Here's the drawing with two shaded views (mm, measured from the low corner). I have some questions. A direction names the side the tool comes from. Round coordinates to 2 decimals unless told otherwise and drop trailing zeros. Loops run counter-clockwise (first coordinate to the right, second up) from the corner with the lowest first, then second, coordinate; pieces in that order, holes last. Notation, with made-up numbers: (25, 59.5) - (75, 59.5) arc R22 cw to (75, 91.5) - close; hole circle Ø2 at (-15, 32). An arc over 180 degrees is marked (long way). Answer as CSV lines item,"result".
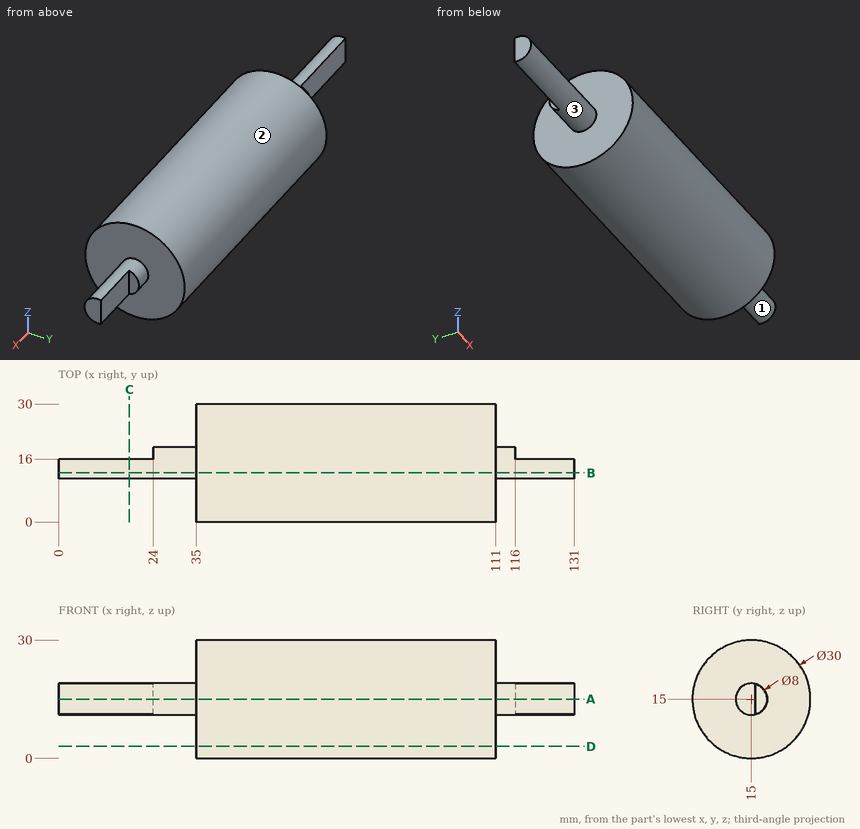
Q1. If I drill on line 1 along X through (y, z) = (7.5, 19.25); line 2 along Y through (x, z) = (103.5, 15.25); line 3 along Z through (x, y) = (8, 14), over which ranges is the centre line in solid material (lowest first)? Write a range as [from, to].
Checks:
line 1,"[35, 111]"
line 2,"[0, 30]"
line 3,"[11.13, 18.87]"
Q2. Imagine slicing it at B-B (y = 12.5). Write out the boundary of the cut face in (x, z).
Checks:
outline,"(0, 11.88) - (35, 11.88) - (35, 0.21) - (111, 0.21) - (111, 11.88) - (131, 11.88) - (131, 18.12) - (111, 18.12) - (111, 29.79) - (35, 29.79) - (35, 18.12) - (0, 18.12) - close"
Q3. Imagine slicing it at A-A (z = 15). Write out the boundary of the cut face in (x, y), then the cut area to 3 significant figures.
Checks:
outline,"(0, 11) - (35, 11) - (35, 0) - (111, 0) - (111, 11) - (131, 11) - (131, 16) - (116, 16) - (116, 19) - (111, 19) - (111, 30) - (35, 30) - (35, 19) - (24, 19) - (24, 16) - (0, 16) - close"
area,"2,600 mm²"
Q4. Imagine slicing it at D-D (z = 3). Write out the boundary of the cut face in (x, y), then the cut area to 3 significant figures.
Checks:
outline,"(35, 6) - (111, 6) - (111, 24) - (35, 24) - close"
area,"1,370 mm²"
Q5. Imagine slicing it at C-C (x = 18). Write out the boundary of the cut face in (y, z).
Checks:
outline,"(16, 11.13) - (16, 18.87) arc R4 ccw (long way) to start"
Q6. On a 3-axis mill with a long thin cutter (end or side, diameter ignored), from which of +Z, -Z, +X, -X, +Y, -Y can I reach the whole of each face in a straight line? I mean the marked faces 1, 2 and 3. Say none if no direction works.
Checks:
face 1,"+X"
face 2,"+X, -X"
face 3,"-X"
Q7. I'm going to push flat-ended pins straight in: pin 1 Ø3 at (y, z) = (17, 27) entering from +X; pin 2 Ø1.5 at (y, z) = (18, 5.5) entering from -X; pin 3 Ø2.5 at (x, z) = (15.5, 16.5) entering from +Y. Where does each tip first touch, or does it pass through?
Checks:
pin 1,"x = 111"
pin 2,"x = 35"
pin 3,"y = 16"
